Part model, mm, in its own coordinate system. A direction names the side the tool comes from. Coordinates: 2 decimals unless noted, no trailing zeros. Order: outer loops, then holes, each group sorted by start corner. A loop starts at its lowest first (then second) coordinate and runs counter-clockwise, first axis right, second up. Notation, with made-up numbers: M 32.5,78.25 L 82.5,78.25 A18 cw 82.5,87.25 Z; hole C 16.25,-11.5 d2. An arc over 180 degrees is marked long. Answer in a Markdown table with one row per item. Add a question column.
from build123d import *

# Parameters (mm, degrees)
BOSS_EXTRUDE1_DEPTH = 3.5
BOSS_EXTRUDE2_DEPTH = 8
FILLET1_R           = 1
SKETCH3_R           = 1.5
CUT_EXTRUDE1_DEPTH  = 8
SKETCH4_R           = 2.5
CUT_EXTRUDE2_DEPTH  = 5
CUT_EXTRUDE3_REACH  = 58.527
SKETCH5_R           = 1.5
SKETCH6_R           = 2.5
CUT_EXTRUDE4_DEPTH  = 5
CUT_EXTRUDE5_REACH  = 57.139
SKETCH7_R           = 1.5
SKETCH8_R           = 6.5
BOSS_EXTRUDE3_DEPTH = 5
CUT_EXTRUDE6_START  = -4
SKETCH9_R           = 6.5
SKETCH9_R_2         = 5.5
CUT_EXTRUDE6_DEPTH  = 3
FILLET2_R           = 1


with BuildPart() as part:
    # Sketch1 → Boss-Extrude1 (new body)
    with BuildSketch(Plane.XY):
        with BuildLine():
            Line((0, 0), (45, 0))
            add(Edge.make_bspline(
                [(45, 0), (45.167594828, -4.342902355), (46.894946491, -9.232868563), (52, -11)],
                knots=[0, 0, 0, 0, 1, 1, 1, 1], degree=3))
            Line((52, -11), (13, -11))
            Line((13, -11), (13, -20.5))
            ThreePointArc((13, -20.5), (6.5, -27), (0, -20.5))
            Line((0, -20.5), (0, 0))
        make_face()
    extrude(amount=BOSS_EXTRUDE1_DEPTH)

    # Sketch2 → Boss-Extrude2 (add)
    with BuildSketch(Plane.XY.offset(3.5)):
        with BuildLine():
            Line((0, 0), (0, -11))
            Line((0, -11), (13, -11))
            Line((13, -11), (52, -11))
            add(Edge.make_bspline(
                [(52, -11), (46.894946491, -9.232868563), (45.167594828, -4.342902355), (45, 0)],
                knots=[0, 0, 0, 0, 1, 1, 1, 1], degree=3))
            Line((45, 0), (0, 0))
        make_face()
    extrude(amount=BOSS_EXTRUDE2_DEPTH)

    # Fillet1
    fillet1_edges = [part.edges().sort_by_distance(p)[0] for p in [
        (52, -11, 7.5),
        (45, 0, 7.5),
        (0, 0, 5.75),
        (0, -11, 7.5),
    ]]
    fillet(fillet1_edges, radius=FILLET1_R)

    # Sketch3 → Cut-Extrude1 (cut)
    with BuildSketch(Plane.XY.offset(3.5)):
        with Locations((9.004616649, -20.5)):
            Circle(SKETCH3_R)
    extrude(amount=-CUT_EXTRUDE1_DEPTH, mode=Mode.SUBTRACT)

    # Sketch4 → Cut-Extrude2 (cut)
    with BuildSketch(Plane.XY.offset(11.5)):
        with Locations((5.5, -5.5)):
            Circle(SKETCH4_R)
    extrude(amount=-CUT_EXTRUDE2_DEPTH, mode=Mode.SUBTRACT)

    # Sketch5 → Cut-Extrude3 (cut, up to next)
    with BuildSketch(Plane.XY.offset(6.5), mode=Mode.PRIVATE) as cut_extrude3_sk1:
        with Locations((5.5, -5.5)):
            Circle(SKETCH5_R)
    cut_extrude3_tool1 = extrude(cut_extrude3_sk1.sketch, amount=-CUT_EXTRUDE3_REACH, mode=Mode.PRIVATE) & part.part
    add(cut_extrude3_tool1.solids().sort_by_distance((5.5, -5.5, 6.5))[0], mode=Mode.SUBTRACT)

    # Sketch6 → Cut-Extrude4 (cut)
    with BuildSketch(Plane(origin=(0, 0, 0), x_dir=(1, 0, 0), z_dir=(0, 1, 0))):
        with Locations(Location((14, -6, 0), (0, 0, 270))):
            Circle(SKETCH6_R)
    extrude(amount=-CUT_EXTRUDE4_DEPTH, mode=Mode.SUBTRACT)

    # Sketch7 → Cut-Extrude5 (cut, up to next)
    with BuildSketch(Plane(origin=(0, -5, 0), x_dir=(1, 0, 0), z_dir=(0, 1, 0)), mode=Mode.PRIVATE) as cut_extrude5_sk1:
        with Locations(Location((14, -6, 0), (0, 0, 270))):
            Circle(SKETCH7_R)
    cut_extrude5_tool1 = extrude(cut_extrude5_sk1.sketch, amount=-CUT_EXTRUDE5_REACH, mode=Mode.PRIVATE) & part.part
    add(cut_extrude5_tool1.solids().sort_by_distance((14, -5, 6))[0], mode=Mode.SUBTRACT)

    # Sketch8 → Boss-Extrude3 (add)
    with BuildSketch(Plane.XY.offset(3.5)):
        with Locations(Location((9.004616649, -20.5, 0), (0, 0, 258.891775774))):
            Circle(SKETCH8_R)
    extrude(amount=BOSS_EXTRUDE3_DEPTH)

    # Sketch9 → Cut-Extrude6 (cut)
    with BuildSketch(Plane.XY.offset(8.5).offset(CUT_EXTRUDE6_START)):
        with Locations(Location((9.004616649, -20.5, 0), (0, 0, 258.891775774))):
            Circle(SKETCH9_R)
        with Locations((9.004616649, -20.5)):
            Circle(SKETCH9_R_2, mode=Mode.SUBTRACT)
    extrude(amount=CUT_EXTRUDE6_DEPTH, mode=Mode.SUBTRACT)

    # Fillet2
    fillet2_edges = [part.edges().sort_by_distance(p)[0] for p in [
        (3.504616649, -20.5, 4.5),
        (3.504616649, -20.5, 7.5),
    ]]
    fillet(fillet2_edges, radius=FILLET2_R - 0.0001)  # a hair under: the kernel refuses the full size


solid = part.part
(1) Wall check: line 1 (Y direction, x = 5.5, z = 7.6); line 2 (Y direction, x = 5.5, z = 4); line 3 (X direction, y = -6.2, z = 6). Give the ranges that are in metal, low to high.
(2) 3-axis set-ups, long thin cutter, end or side, ignore diameter. For faces 5 (the flat face through (14, -22, 3.5)), 6 (the flat face through (12, -5, 6)), 7 (the cylindrical face through (10.536, -14.183, 7.993)): which of +Z, -Z, +X, -X, +Y, -Y reach the whole face in a straight line?
(3) Slice it at B-B (x = 20.5). List the corners of the cut face in (y, z), and give its area (4 significant figures).
(4) Slice it at A-A (z = 6). State how many separate pieces and enclosed holes the cut face has, and give its area (3 significant figures).
(5) Pull direction Y, two halves, no side cores. Call faces 1 (the cylindrical face through (0.285, -10.699, 7.556)), 2 (the flat face through (9, -20, 3.5)), 3 (the flat face through (19, -7, 0)), 4 (the flat face through (23, 0, 6)): pulls with the +Y half, pulls with the -Y half, needs draft (parallel to the pull), parting line crosses it, or undercut.
(6) Drop flat-ended pins along their axis: P1, Ø14.5, axis at x = 9.5, y = -22, coming from the +Z side; P2, Ø3.5, axis at x = 14, z = 6, coming from the -Y side; P3, Ø3.5, axis at x = 5.5, y = -5.5, coming from the +Z side; P4, Ø5, axis at x = 9, y = -20.5, coming from the -Z side. Give the stop position or say it passes through.
Computed:
| question | item | result |
|---|---|---|
| 1 | line 1 | y = -25.97 to -15.03, -11 to -8, -3 to 0 |
| 1 | line 2 | y = -25.97 to -15.03, -11 to -7, -4 to 0 |
| 1 | line 3 | x = 0 to 4.17, 6.83 to 12.5, 15.5 to 46.51 |
| 2 | face 5 | -Z, +X, -Y |
| 2 | face 6 | +Y |
| 2 | face 7 | +Z |
| 3 | outline | M -11,0 L 0,0 L 0,11.5 L -11,11.5 Z |
| 3 | area | 126.5 mm^2 |
| 4 | separate pieces | 3 |
| 4 | enclosed holes | 1 |
| 4 | area | 557 mm^2 |
| 5 | face 1 | pulls with the -Y half |
| 5 | face 2 | undercut |
| 5 | face 3 | needs draft |
| 5 | face 4 | pulls with the +Y half |
| 6 | P1 | stops at z = 8.5 |
| 6 | P2 | stops at y = -25.55 |
| 6 | P3 | stops at z = 6.5 |
| 6 | P4 | stops at z = 0 |
